```python
from build123d import *


# Not quite as in the source:
# - a feature of the source that left no trace in its solid (it failed there, or was rolled back) is left out
# - a feature names something its author has since deleted; it is built from what else it names


with BuildPart() as f1:
    # F0 (on Front) → F1 (revolve)
    with BuildSketch(Plane.XZ):
        with BuildLine():
            ThreePointArc((10.9666396311, 27.1683829889), (12.4701625396, 28.6523491091), (10.9666396311, 30.1363152292))
            ThreePointArc((10.9666396311, 30.1363152292), (3.1518347441, 26.8641196143), (0, 19))
            Line((0, 19), (0.0767615013, 14.0005892675))
            Line((0.0767615013, 14.0005892675), (2.9666396311, 14.0449607736))
            Line((2.9666396311, 14.0449607736), (2.9666396311, 4.1683829889))
            Line((2.9666396311, 4.1683829889), (5.9666396311, 4.1683829889))
            Line((5.9666396311, 4.1683829889), (5.9666396311, 14.1683829889))
            ThreePointArc((5.9666396311, 14.1683829889), (3.7741797187, 16.2529070415), (2.9666396311, 19.1683829889))
            ThreePointArc((2.9666396311, 19.1683829889), (5.3097853816, 24.8252372384), (10.9666396311, 27.1683829889))
        make_face()
    revolve(axis=Axis((-15, 0, 28.4551028162), (0, 0, 1)))


solid = f1.part
```
Geometry check sheet. Reference: the model listing, model coordinates, mm. Give positions to 0.01 mm unless a question says otherwise; leave off trailing zeros. Loops run counter-clockwise (first coordinate to the right, second up) from the corner with the lowest first, then second, coordinate; pieces in that order, holes last. Notation, with made-up numbers: M 5,-17.75 L 28,-17.75 A27 cw 28,11.25 Z; hole C 83.25,87.25 d9. An arc over 180 degrees is marked long. Write item = value, one per line.
(1) Gauge pin test, flat ends, axial feed: pin 1 Ø10 at (x, z) = (-27.5, 15.5) entering from -Y; pin 2 Ø1.5 at (y, z) = (4.5, 13) entering from -X; pin 3 Ø1 at (x, z) = (-13, 12) entering from -Y; pin 4 Ø8 at (x, y) = (-18, 8.5) entering from +Z. Record the tip position at first contact, or that the pin passes through.
Answer below:
pin_1 = -19.51
pin_2 = -35.63
pin_3 = -20.91
pin_4 = through
(2) Sectioned sample at B-B, the plane z = 21. Record the cut outline in (x, y).
Answer below:
outline = C -15,0 d36.36; hole C -15,0 d30.31
(3) Release check for a two-part mould opening along Y. For faces 1 (the face through (-32.95, 0.79, 9.04)), 2 (the face through (-30.243, 0.671, 14.003)), 3 (the face through (-32, 6.3, 4.168)), 4 (the face through (4.37, -8.03, 9.24)) record: released by +Y, released by -Y, zero draft, split by the parting line, or undercut.
Answer below:
face_1 = undercut
face_2 = undercut
face_3 = zero draft
face_4 = split by the parting line
(4) Material ranges on line 1 (Y direction, x = -15, z = 8.25); line 2 (X direction, y = 1, z = 7); line 3 (X direction, y = 4.5, z = 17.25), recorded low to high. Write a range as [from, to].
Answer below:
line_1 = [-20.97, -17.97], [17.97, 20.97]
line_2 = [-35.94, -32.94], [2.94, 5.94]
line_3 = [-32.74, -29.34], [-0.66, 2.74]
(5) Sectioned sample at A-A, the plane z = 7.75. Record the cut outline in (x, y).
Answer below:
outline = C -15,0 d41.93; hole C -15,0 d35.93
